```python
from build123d import *

# Parameters (mm, degrees)
SKETCH_1_R             = 7
SM_BASE_FLANGE_1_DEPTH = 4


# Sheet-metal steps are written as plain solids
with BuildPart() as part:
    # Sketch 1 → Базовая кромка1 (new body)
    with BuildSketch(Plane(origin=(0, 0, 0), x_dir=(0, 0, -1), z_dir=(1, 0, 0))):
        with BuildLine():
            Line((0, 20), (305, 20))
            ThreePointArc((305, 20), (325, 0), (305, -20))
            Line((305, -20), (0, -20))
            ThreePointArc((0, -20), (-20, 0), (0, 20))
        make_face()
        Circle(SKETCH_1_R, mode=Mode.SUBTRACT)
        with Locations((305, 0)):
            Circle(SKETCH_1_R, mode=Mode.SUBTRACT)
        with Locations((170, 0)):
            Circle(SKETCH_1_R, mode=Mode.SUBTRACT)
    extrude(amount=-SM_BASE_FLANGE_1_DEPTH)


solid = part.part
```
CAD build for the part. Positions are in the model's coordinates, mm. Give positions to 0.01 mm unless a question says otherwise; leave off trailing zeros. Order: outer loops, then holes, each group sorted by start corner. A loop starts at its lowest first (then second) coordinate and runs counter-clockwise, first axis right, second up.
(1) Saw through at C-C, the plane z = -170. Give the cut face in (x, y).
(2) Saw through at A-A, the plane y = 0. Give the cut face in (x, z), then the cut area to 3 significant figures.
(3) Mould opens along Z. For faces 1 (the cylindrical face through (-1.972, -2.681, -6.466)), 2 (the cylindrical face through (-1.972, -2.681, -176.466)), 3 (the cylindrical face through (-2, 0, -325)), 4 (the cylindrical face through (-2, 0, 20)) say: released by +Z, released by -Z, zero draft, split by the parting line, or undercut.
(4) Saw through at B-B, the plane x = -0.9. Give the cut face in (y, z), then the cut area to 3 significant figures.
(5) Drill centre lines: L1, parallel to Y at x = -1.5, z = -170; L2, parallel to Z at x = -1.35, y = -0.5; L3, parallel to Z at x = -2.1, y = 1. Where is each one in solid material? Low to high.
(6) Flat gauge pin, fed straight in: pin 1 (2 mm diameter, centred on x = -2.5, y = -6.5, fed in from -Z). Where does the tip first touch, or does it go through?
(7) Saw through at D-D, the plane y = 15. Give the cut face in (x, z).
Results found:
1. outline: (-4, -20) - (0, -20) - (0, -7) - (-4, -7) - close; (-4, 7) - (0, 7) - (0, 20) - (-4, 20) - close
2. outline: (-4, -325) - (0, -325) - (0, -312) - (-4, -312) - close; (-4, -298) - (0, -298) - (0, -177) - (-4, -177) - close; (-4, -163) - (0, -163) - (0, -7) - (-4, -7) - close; (-4, 7) - (0, 7) - (0, 20) - (-4, 20) - close
2. area: 1,210 mm2
3. face 1: undercut
3. face 2: undercut
3. face 3: released by -Z
3. face 4: released by +Z
4. outline: (-20, -305) arc R20 ccw to (20, -305) - (20, 0) arc R20 ccw to (-20, 0) - close; hole circle Ø14 at (0, -305); hole circle Ø14 at (0, -170); hole circle Ø14 at (0, 0)
4. area: 13,000 mm2
5. L1: y = -20 to -7, 7 to 20
5. L2: z = -324.99 to -311.98, -298.02 to -176.98, -163.02 to -6.98, 6.98 to 19.99
5. L3: z = -324.97 to -311.93, -298.07 to -176.93, -163.07 to -6.93, 6.93 to 19.97
6. pin 1: stops at z = -324.23
7. outline: (-4, -318.23) - (0, -318.23) - (0, 13.23) - (-4, 13.23) - close
